Part model, mm, in its own coordinate system. A direction names the side the tool comes from. Give positions to 0.01 mm unless a question says otherwise; leave off trailing zeros. Order: outer loops, then holes, each group sorted by start corner. A loop starts at its lowest first (then second) coordinate and runs counter-clockwise, first axis right, second up. Notation, with made-up numbers: M 2.5,84.25 L 7.5,84.25 A11 cw 7.5,105.25 Z; hole C -32,-15.5 d8. An arc over 180 degrees is marked long. Write each question's results on one line, items separated by ' | '. Start each with the question number.
Autodesk Inventor part; units mm, degrees
ref_plane "YZ Plane" through (0, 0, 0) normal (1, 0, 0) x (0, 1, 0)
ref_plane "XZ Plane" through (0, 0, 0) normal (0, 1, 0) x (-1, 0, 0)
ref_plane "XY Plane" through (0, 0, 0) normal (0, 0, 1) x (1, 0, 0)
sketch "Sketch1" plane through (0, 0, 0) normal (0, 1, 0) x (-1, 0, 0)
  line L0 (-39, -24.5) -> (19, -24.5) construction
  line L1 (19, -24.5) -> (19, 24.5) construction
  line L2 (19, 24.5) -> (-39, 24.5) construction
  line L3 (-39, 24.5) -> (-39, -24.5) construction
  line L4 (42.5, -28) -> (-42.5, -28) construction
  line L5 (-42.5, -28) -> (-42.5, 28) construction
  line L6 (-42.5, 28) -> (42.5, 28) construction
  line L7 (42.5, 28) -> (42.5, -28) construction
  line L8 (50, 0) -> (-50, 0) construction
  line L9 (47.5, -33) -> (-47.5, -33) construction
  line L10 (-47.5, -33) -> (-47.5, 33) construction
  line L11 (-47.5, 33) -> (47.5, 33) construction
  line L12 (47.5, 33) -> (47.5, -33) construction
  circle A0 centre (47.5, -33) radius 7.5
  circle A1 centre (47.5, 33) radius 7.5
  circle A2 centre (-47.5, 33) radius 7.5
  circle A3 centre (-47.5, -33) radius 7.5
  line L13 (49.5, -25.7716) -> (49.5, 25.7716)
  line L14 (40.2716, 35) -> (-40.2716, 35)
  line L15 (-49.5, 25.7716) -> (-49.5, -25.7716)
  line L16 (-40.2716, -35) -> (40.2716, -35)
  arc A4 (-49.5, -15) -> (-49.5, 15) centre (-59.5625, 0) ccw
  point P0 (0, 0)
  point P1 (-39, 0)
  point P2 (0, 0)
  point P3 (0, -28)
  point P4 (0, 0)
  point P5 (0, -33)
  point P6 (-47.5, 0)
  point P7 (-41.5, 0)
  dimension "d0" = 58
  dimension "d1" = 49
  dimension "d2" = 3.5
  dimension "d3" = 3.5
  dimension "d25" = 5
  dimension "d26" = 5
  dimension "d27" = 15
  dimension "d28" = 85
  dimension "d29" = 2
  dimension "d30" = 2
  dimension "d32" = 30
  dimension "d33" = 8
extrude "Extrusion1" add sketch "Sketch1" along normal blind 3 contours A0 | A0 L16 A3 L15 A4 A2 L14 A1 L13 | A1 | A3 | A2
fillet "Fillet2" radius 8 8 edges at (-49.5, 1.5, -25.7716) (-49.5, 1.5, 25.7716) (-40.2716, 1.5, 35) (40.2716, 1.5, 35) (49.5, 1.5, 25.7716) (49.5, 1.5, -25.7716) (40.2716, 1.5, -35) (-40.2716, 1.5, -35)
hole "Hole1" at (-47.5, 0, 33) at (-47.5, 0, -33) at (47.5, 0, -33) at (47.5, 0, 33) direction (0, 1, 0) diameter 3 end through all
hole "Hole2" at (-19, 0, 24.5) at (-19, 0, -24.5) at (39, 0, -24.5) at (39, 0, 24.5) direction (0, 1, 0) diameter 2.5 end through all
sketch "Sketch3" plane through (0, 3, 0) normal (0, 1, 0) x (1, 0, 0)
  circle A0 centre (39, 24.5) radius 1.25
  circle A1 centre (-19, -24.5) radius 1.25
  circle A2 centre (-19, 24.5) radius 1.25
  circle A3 centre (39, -24.5) radius 1.25
  circle A4 centre (47.5, 33) radius 1.5
  circle A5 centre (-47.5, -33) radius 1.5
  circle A6 centre (-47.5, 33) radius 1.5
  circle A7 centre (47.5, -33) radius 1.5
  line L0 (49.5, 15) -> (49.5, 21.1573)
  arc A8 (52.3387, 27.2697) -> (49.5, 21.1573) centre (57.5, 21.1573) ccw
  arc A9 (52.3387, 27.2697) -> (41.7697, 37.8387) centre (47.5, 33) ccw
  arc A10 (35.6573, 35) -> (41.7697, 37.8387) centre (35.6573, 43) ccw
  line L1 (35.6573, 35) -> (-35.6573, 35)
  arc A11 (-41.7697, 37.8387) -> (-35.6573, 35) centre (-35.6573, 43) ccw
  arc A12 (-41.7697, 37.8387) -> (-52.3387, 27.2697) centre (-47.5, 33) ccw
  arc A13 (-49.5, 21.1573) -> (-52.3387, 27.2697) centre (-57.5, 21.1573) ccw
  line L2 (-49.5, 21.1573) -> (-49.5, -21.1573)
  arc A14 (-52.3387, -27.2697) -> (-49.5, -21.1573) centre (-57.5, -21.1573) ccw
  arc A15 (-52.3387, -27.2697) -> (-41.7697, -37.8387) centre (-47.5, -33) ccw
  arc A16 (-35.6573, -35) -> (-41.7697, -37.8387) centre (-35.6573, -43) ccw
  line L3 (-35.6573, -35) -> (35.6573, -35)
  arc A17 (41.7697, -37.8387) -> (35.6573, -35) centre (35.6573, -43) ccw
  arc A18 (41.7697, -37.8387) -> (52.3387, -27.2697) centre (47.5, -33) ccw
  arc A19 (49.5, -21.1573) -> (52.3387, -27.2697) centre (57.5, -21.1573) ccw
  line L4 (49.5, -21.1573) -> (49.5, -15)
  arc A20 (49.5, 15) -> (49.5, -15) centre (59.5625, 0) ccw
  point P0 (0, 0)
equation "\"d3\" = d2"
equation "\"d26\" = d25"
equation "\"d30\" = d29"
properties part number "plate_mounting"
(1) Drop a flat-ended pin along its axis: P1, Ø1.5, axis at x = 39, z = 24.5, coming from the +Y side. Give the stop position or say it passes through.
(2) Tool access for faces 5 (the flat face through (49.5, 1, 18)), 6 (the cylindrical face through (-50.265, 1.521, 24.571)), 7 (the flat face through (0, 1, 35)): list every direction of +Z, -Z, +X, -X, +Y, -Y with a clear straight run to the whole face (end or side of a thin tool).
(3) Pull direction Z, two halves, no side cores. Call faces 1 (the cylindrical face through (39.479, 1.521, -25.655)), 2 (the cylindrical face through (-38.983, 1.521, 35.724)), 3 (the cylindrical face through (-52.925, 1.479, -38.179)), 4 (the cylindrical face through (38.983, 1.521, -35.724)): +Z half, -Z half, draft (parallel to the pull), parting line (faces both ways), or undercut.
(4) Probe L1, parallel to X at y = 1.9, z = -33; L2, parallel to Z at x = -19, y = 1.2; L3, parallel to X at y = 0.8, z = -32.5. List the from-to ranges inside material, lowest first.
(5) Saw through at B-B on z = 33. Give the cut face in (x, y).
(6) Saw through at D-D on x = 47.5. Give the cut face in (y, z), plus the area to 3 significant figures.
(7) Saw through at C-C on y = 2.5. Give the number of separate pieces and of enclosed holes in the cut face, plus the area to 3 significant figures.
(8) Saw through at A-A on x = -47.5. Give the cut face in (y, z), plus the area to 3 significant figures.
Taken from the geometry:
1) P1: passes through
2) face 5: +X, +Y, -Y | face 6: -X, +Y, -Y | face 7: +Z, +Y, -Y
3) face 1: undercut | face 2: +Z half | face 3: undercut | face 4: -Z half
4) L1: x = -55 to -49, -46 to 46, 49 to 55 | L2: z = -35 to -25.75, -23.25 to 23.25, 25.75 to 35 | L3: x = -54.98 to -48.91, -46.09 to 46.09, 48.91 to 54.98
5) outline: M -55,0 L -49,0 L -49,3 L -55,3 Z; M -46,0 L 46,0 L 46,3 L -46,3 Z; M 49,0 L 55,0 L 55,3 L 49,3 Z
6) outline: M 0,-40.5 L 3,-40.5 L 3,-34.5 L 0,-34.5 Z; M 0,-31.5 L 3,-31.5 L 3,-13.44 L 0,-13.44 Z; M 0,13.44 L 3,13.44 L 3,31.5 L 0,31.5 Z; M 0,34.5 L 3,34.5 L 3,40.5 L 0,40.5 Z | area: 144 mm²
7) separate pieces: 1 | enclosed holes: 8 | area: 7,130 mm²
8) outline: M 0,-40.5 L 3,-40.5 L 3,-34.5 L 0,-34.5 Z; M 0,-31.5 L 3,-31.5 L 3,31.5 L 0,31.5 Z; M 0,34.5 L 3,34.5 L 3,40.5 L 0,40.5 Z | area: 225 mm²
